from build123d import *

# Parameters (mm, degrees)
SKETCH1_R           = 1.25
BOSS_EXTRUDE1_DEPTH = 166.878


with BuildPart() as part:
    # Sketch1 → Boss-Extrude1 (new body)
    with BuildSketch(Plane.XY.offset(300)):
        with BuildLine():
            Line((-7.5, 6.5), (-7.5, 2))
            ThreePointArc((-7.5, 2), (-7.412132034, 1.787867966), (-7.2, 1.7))
            Line((-7.2, 1.7), (-6.4, 1.7))
            Line((-6.4, 1.7), (-6.4, 2.85))
            Line((-6.4, 2.85), (-3.8, 2.85))
            Line((-3.8, 2.85), (-2.8, 1.85))
            Line((-2.8, 1.85), (-2.8, 0.519615242))
            Line((-2.8, 0.519615242), (-2.5, 0))
            Line((-2.5, 0), (-2.8, -0.519615242))
            Line((-2.8, -0.519615242), (-2.8, -1.85))
            Line((-2.8, -1.85), (-3.8, -2.85))
            Line((-3.8, -2.85), (-6.4, -2.85))
            Line((-6.4, -2.85), (-6.4, -1.7))
            Line((-6.4, -1.7), (-7.2, -1.7))
            ThreePointArc((-7.2, -1.7), (-7.412132034, -1.787867966), (-7.5, -2))
            Line((-7.5, -2), (-7.5, -6.5))
            ThreePointArc((-7.5, -6.5), (-7.207106781, -7.207106781), (-6.5, -7.5))
            Line((-6.5, -7.5), (-2, -7.5))
            ThreePointArc((-2, -7.5), (-1.787867966, -7.412132034), (-1.7, -7.2))
            Line((-1.7, -7.2), (-1.7, -6.4))
            Line((-1.7, -6.4), (-2.85, -6.4))
            Line((-2.85, -6.4), (-2.85, -3.8))
            Line((-2.85, -3.8), (-1.85, -2.8))
            Line((-1.85, -2.8), (-0.519615242, -2.8))
            Line((-0.519615242, -2.8), (0, -2.5))
            Line((0, -2.5), (0.519615242, -2.8))
            Line((0.519615242, -2.8), (1.85, -2.8))
            Line((1.85, -2.8), (2.85, -3.8))
            Line((2.85, -3.8), (2.85, -6.4))
            Line((2.85, -6.4), (1.7, -6.4))
            Line((1.7, -6.4), (1.7, -7.2))
            ThreePointArc((1.7, -7.2), (1.787867966, -7.412132034), (2, -7.5))
            Line((2, -7.5), (6.5, -7.5))
            ThreePointArc((6.5, -7.5), (7.207106781, -7.207106781), (7.5, -6.5))
            Line((7.5, -6.5), (7.5, -2))
            ThreePointArc((7.5, -2), (7.412132034, -1.787867966), (7.2, -1.7))
            Line((7.2, -1.7), (6.4, -1.7))
            Line((6.4, -1.7), (6.4, -2.85))
            Line((6.4, -2.85), (3.8, -2.85))
            Line((3.8, -2.85), (2.8, -1.85))
            Line((2.8, -1.85), (2.8, -0.519615242))
            Line((2.8, -0.519615242), (2.5, 0))
            Line((2.5, 0), (2.8, 0.519615242))
            Line((2.8, 0.519615242), (2.8, 1.85))
            Line((2.8, 1.85), (3.8, 2.85))
            Line((3.8, 2.85), (6.4, 2.85))
            Line((6.4, 2.85), (6.4, 1.7))
            Line((6.4, 1.7), (7.2, 1.7))
            ThreePointArc((7.2, 1.7), (7.412132034, 1.787867966), (7.5, 2))
            Line((7.5, 2), (7.5, 6.5))
            ThreePointArc((7.5, 6.5), (7.207106781, 7.207106781), (6.5, 7.5))
            Line((6.5, 7.5), (2, 7.5))
            ThreePointArc((2, 7.5), (1.787867966, 7.412132034), (1.7, 7.2))
            Line((1.7, 7.2), (1.7, 6.4))
            Line((1.7, 6.4), (2.85, 6.4))
            Line((2.85, 6.4), (2.85, 3.8))
            Line((2.85, 3.8), (1.85, 2.8))
            Line((1.85, 2.8), (0.519615242, 2.8))
            Line((0.519615242, 2.8), (0, 2.5))
            Line((0, 2.5), (-0.519615242, 2.8))
            Line((-0.519615242, 2.8), (-1.85, 2.8))
            Line((-1.85, 2.8), (-2.85, 3.8))
            Line((-2.85, 3.8), (-2.85, 6.4))
            Line((-2.85, 6.4), (-1.7, 6.4))
            Line((-1.7, 6.4), (-1.7, 7.2))
            ThreePointArc((-1.7, 7.2), (-1.787867966, 7.412132034), (-2, 7.5))
            Line((-2, 7.5), (-6.5, 7.5))
            ThreePointArc((-6.5, 7.5), (-7.207106781, 7.207106781), (-7.5, 6.5))
        make_face()
        with Locations(Location((0, 0, 0), (0, 0, 180))):
            Circle(SKETCH1_R, mode=Mode.SUBTRACT)
    extrude(amount=-BOSS_EXTRUDE1_DEPTH)


solid = part.part
Geometry check sheet. Reference: the model listing, model coordinates, mm. A direction names the side the tool comes from. Round coordinates to 2 decimals unless told otherwise and drop trailing zeros. Answer as a JSON object with one key per item and string values. Group by question number.
Item 1: Release check for a two-part mould opening along X. For faces 3 (the face through (7.5, 4, 218)), 4 (the face through (2.85, 5, 218)), 5 (the face through (-4, -7.5, 218)) record: pulls with the +X half, pulls with the -X half, needs draft (parallel to the pull), parting line crosses it, or undercut.
Item 2: Set-up check for faces 1 (the face through (5, 2.85, 218)), 2 (the face through (-4, 7.5, 218)): record each of +Z, -Z, +X, -X, +Y, -Y from which the full face is reachable in a straight line by a thin tool's end or side.
Item 3: Depth check by flat-ended pin: pin 1 Ø0.6 at (x, z) = (-7, 215.5) entering from -Y; pin 2 Ø1.1 at (x, z) = (1, 209) entering from -Y; pin 3 Ø1 at (y, z) = (-1, 184.5) entering from +X. Enter the tip coordinate at first touch or a pass-through.
Item 4: Thickness scan on line 1 along Y through (x, z) = (-5, 152); line 2 along Y through (x, z) = (0, 167.5). Record the ranges inside material, lowest first.
Determined:
{
 "1": {"face 3": "pulls with the +X half", "face 4": "undercut", "face 5": "needs draft"},
 "2": {"face 1": "+Z, -Z", "face 2": "+Z, -Z, +X, -X, +Y"},
 "3": {"pin 1": "stops at y = -7.48", "pin 2": "stops at y = -2.8", "pin 3": "stops at x = 2.8"},
 "4": {"line 1": "y = -7.5 to -2.85, 2.85 to 7.5", "line 2": "y = -2.5 to -1.25, 1.25 to 2.5"}
}
